from build123d import *


with BuildPart() as part:
    # Sketch1 → Revolve1 (revolve)
    with BuildSketch(Plane.XY, mode=Mode.PRIVATE) as revolve1_sk:
        with BuildLine():
            Line((-3.95, 1.25), (3.95, 1.25))
            Line((3.95, 1.25), (3.95, 1))
            Line((3.95, 1), (4.55, 1))
            Line((4.55, 1), (4.675, 1.125))
            Line((4.675, 1.125), (4.851776695, 0.948223305))
            Line((4.851776695, 0.948223305), (4.726776695, 0.823223305))
            ThreePointArc((4.726776695, 0.823223305), (4.645670858, 0.769030117), (4.55, 0.75))
            Line((4.55, 0.75), (-4.55, 0.75))
            ThreePointArc((-4.55, 0.75), (-4.645670858, 0.769030117), (-4.726776695, 0.823223305))
            Line((-4.726776695, 0.823223305), (-4.851776695, 0.948223305))
            Line((-4.851776695, 0.948223305), (-4.675, 1.125))
            Line((-4.675, 1.125), (-4.55, 1))
            Line((-4.55, 1), (-3.95, 1))
            Line((-3.95, 1), (-3.95, 1.25))
        make_face()
    revolve(revolve1_sk.sketch.rotate(Axis((-108.445306304, 0, 0), (1, 0, 0)), 90), axis=Axis((-108.445306304, 0, 0), (1, 0, 0)))


solid = part.part
Could you check a few things on this model? Use its own coordinates, in mm. A direction names the side the tool comes from. Give positions to 0.01 mm unless a question says otherwise; leave off trailing zeros. Order: outer loops, then holes, each group sorted by start corner. A loop starts at its lowest first (then second) coordinate and runs counter-clockwise, first axis right, second up.
1. I need wall thicknesses on L1, parallel to Y at x = -2.5, z = 0; L2, parallel to Z at x = 4.5, y = 0.05. Which ranges of each line are inside material? Lowest first, please.
Answers below:
L1: y = -1.25 to -0.75, 0.75 to 1.25
L2: z = -1 to -0.75, 0.75 to 1
2. Suppose I cut it at A-A (z = 0). Write out the boundary of the cut face in (x, y) (3 decimals), plus the area to 3 significant figures.
Answers below:
outline: (-4.852, -0.948) - (-4.675, -1.125) - (-4.55, -1) - (-3.95, -1) - (-3.95, -1.25) - (3.95, -1.25) - (3.95, -1) - (4.55, -1) - (4.675, -1.125) - (4.852, -0.948) - (4.727, -0.823) arc R0.25 ccw to (4.55, -0.75) - (-4.55, -0.75) arc R0.25 ccw to (-4.727, -0.823) - close; (-4.852, 0.948) - (-4.727, 0.823) arc R0.25 ccw to (-4.55, 0.75) - (4.55, 0.75) arc R0.25 ccw to (4.727, 0.823) - (4.852, 0.948) - (4.675, 1.125) - (4.55, 1) - (3.95, 1) - (3.95, 1.25) - (-3.95, 1.25) - (-3.95, 1) - (-4.55, 1) - (-4.675, 1.125) - close
area: 8.77 mm2
3. Suppose I cut it at C-C (x = -2). Write out the boundary of the cut face in (y, z), plus the area to 3 significant figures.
Answers below:
outline: circle Ø2.5 at (0, 0); hole circle Ø1.5 at (0, 0)
area: 3.14 mm2
4. Which directions (+Z, -Z, +X, -X, +Y, -Y) give clear straight access to the entire face, cutting with the end or side of a thin tool? Please do faces 1 (the cylindrical face through (0.06, -0.05, -1.25)), 2 (the cylindrical face through (4.254, 0.976, -0.217)).
Answers below:
face 1: +X, -X
face 2: none
5. Thinking about a two-plate mould opening in Z: for faces 3 (the cylindrical face through (-4.246, 0.976, -0.217)), 4 (the cylindrical face through (-0.064, -0.225, 0.715)), which applies, +Z half, -Z half, draft (parallel to the pull), parting line (faces both ways), or undercut?
Answers below:
face 3: parting line
face 4: undercut
